from build123d import *

# Parameters (mm, degrees)
F1_DEPTH = 25.4
F2_W     = 8.4582
F2_H     = 8.4709
F3_DEPTH = 25.4


with BuildPart() as f1:
    # F0 (on Front) → F1 (new body)
    with BuildSketch(Plane.XZ):
        Polygon((-25.4, 0), (0, 0), (0, 25.4), (-8.4836, 25.4), (-8.4836, 16.9418), (-25.4, 16.9418), align=None)
    extrude(amount=F1_DEPTH)

    # F2 (on face) → F3 (cut)
    with BuildSketch(Plane.XZ.offset(25.4)):
        with Locations((-21.1709, 12.70635)):
            Rectangle(F2_W, F2_H)
    extrude(amount=-F3_DEPTH, mode=Mode.SUBTRACT)


solid = f1.part
Work out the finished part from the listing and answer in its coordinate system (mm). A direction names the side the tool comes from. Round coordinates to 2 decimals unless told otherwise and drop trailing zeros. Write each loop counter-clockwise with the first axis right and the second up, starting at its lowest first coordinate (ties: lowest second). Pieces come first, ordered by that corner, then holes.
1) A cutting plane is placed at C-C (z = 23.25). Give the vertices of the cut face in (x, y), plus the area to 3 significant figures.
2) Given pin 1 Ø1.5 at (y, z) = (-3, 22.5) entering from -X; pin 2 Ø4 at (x, y) = (-22.5, -18.5) entering from +Z; pin 3 Ø2.5 at (x, y) = (-12, -8) entering from +Z, each flat-ended and moving along its own axis, determine where each tip first touches the part or whether it passes through.
3) A tool of negligible diameter and unlimited length cuts with its end or side. For faces 1 (the flat face through (-10, 0, 10)), 2 (the flat face through (-13, -13, 16.942)), from which of +Z, -Z, +X, -X, +Y, -Y can it reach the whole face along a straight path? Write none if from no direction.
4) A cutting plane is placed at A-A (y = -18.5). Give the vertices of the cut face in (x, z), plus the area to 3 significant figures.
5) Straight lines are drawn through the part: line 1 (X direction, y = -12, z = 11.75); line 2 (X direction, y = -5.75, z = 19.5); line 3 (Z direction, x = -8.75, y = -3). For each, find the intervals that lie inside material, in ascending order.
6) A cutting plane is placed at B-B (x = -17.5). Give the vertices of the cut face in (y, z), plus the area to 3 significant figures.
Completed:
1. outline: (-8.48, -25.4) - (0, -25.4) - (0, 0) - (-8.48, 0) - close
1. area: 215 mm2
2. pin 1: stops at x = -8.48
2. pin 2: stops at z = 8.47
2. pin 3: stops at z = 16.94
3. face 1: +Z, -Z, +X, -X, +Y
3. face 2: +Z, -X, +Y, -Y
4. outline: (-25.4, 0) - (0, 0) - (0, 25.4) - (-8.48, 25.4) - (-8.48, 16.94) - (-16.94, 16.94) - (-16.94, 8.47) - (-25.4, 8.47) - close
4. area: 430 mm2
5. line 1: x = -16.94 to 0
5. line 2: x = -8.48 to 0
5. line 3: z = 0 to 16.94
6. outline: (-25.4, 0) - (0, 0) - (0, 8.47) - (-25.4, 8.47) - close
6. area: 215 mm2
